Autodesk Inventor part; units mm, degrees
ref_plane "YZ Plane" through (0, 0, 0) normal (1, 0, 0) x (0, 1, 0)
ref_plane "XZ Plane" through (0, 0, 0) normal (0, 1, 0) x (-1, 0, 0)
ref_plane "XY Plane" through (0, 0, 0) normal (0, 0, 1) x (1, 0, 0)
sketch "Sketch1" plane through (0, 0, 0) normal (0, 0, 1) x (1, 0, 0)
  line L0 (0, 0) -> (22.5, 0)
  line L1 (22.5, 0) -> (22.5, 22.5)
  line L2 (22.5, 22.5) -> (0, 22.5)
  line L3 (0, 22.5) -> (0, 0)
  line L4 (0, 0) -> (20.5, 0)
  line L5 (20.5, 0) -> (20.5, 2)
  line L6 (20.5, 2) -> (0, 2)
  line L7 (0, 2) -> (0, 0)
  line L8 (22.5, 0) -> (20.5, 0)
  line L9 (20.5, 0) -> (20.5, 20.5)
  line L10 (20.5, 20.5) -> (22.5, 20.5)
  line L11 (22.5, 20.5) -> (22.5, 0)
  line L12 (22.5, 22.5) -> (2, 22.5)
  line L13 (2, 22.5) -> (2, 20.5)
  line L14 (2, 20.5) -> (22.5, 20.5)
  line L15 (22.5, 20.5) -> (22.5, 22.5)
  line L16 (0, 22.5) -> (2, 22.5)
  line L17 (2, 22.5) -> (2, 2)
  line L18 (2, 2) -> (0, 2)
  line L19 (0, 2) -> (0, 22.5)
  line L20 (2, 2) -> (20.5, 2)
  line L21 (20.5, 2) -> (20.5, 20.5)
  line L22 (20.5, 20.5) -> (2, 20.5)
  line L23 (2, 20.5) -> (2, 2)
  dimension "d0" = 22.5
  dimension "d1" = 22.5
  dimension "d2" = 20.5
  dimension "d3" = 2
  dimension "d4" = 2
  dimension "d5" = 20.5
  dimension "d6" = 20.5
  dimension "d7" = 2
  dimension "d8" = 2
  dimension "d9" = 20.5
  dimension "d10" = 18.5
  dimension "d11" = 18.5
extrude "Extrusion1" add sketch "Sketch1" along normal blind 69
sketch "Sketch2" plane through (0, 0, 0) normal (0, -1, 0) x (1, 0, 0)
  line L0 (0, 69) -> (22.5, 69)
  line L1 (22.5, 69) -> (20.5, 69)
  line L2 (20.5, 69) -> (20.5, 2)
  line L3 (20.5, 2) -> (22.5, 2)
  line L4 (22.5, 2) -> (22.5, 69)
  line L5 (20.5, 2) -> (2, 2)
  line L6 (2, 2) -> (2, 68)
  line L7 (2, 68) -> (20.5, 68)
  line L8 (20.5, 68) -> (20.5, 2)
  point P0 (0, 0)
  dimension "d14" = 2
  dimension "d15" = 67
  dimension "d16" = 18.5
  dimension "d17" = 66
extrude "Extrusion2" cut sketch "Sketch2" against normal blind 18.5 contours L2 L5 L6 L7
sketch "Sketch3" plane through (0, 0, 69) normal (0, 0, 1) x (1, 0, 0)
  line L0 (22.5, 22.5) -> (0, 22.5)
  line L1 (0, 0) -> (22.5, 0)
  line L2 (0, 22.5) -> (22.5, 22.5)
  line L3 (22.5, 22.5) -> (22.5, 0)
  line L4 (22.5, 0) -> (0, 0)
  line L5 (0, 0) -> (0, 22.5)
  dimension "d20" = 22.5
  dimension "d21" = 22.5
extrude "Extrusion3" add sketch "Sketch3" along normal blind 1
sketch "Sketch4" plane through (0, 18.5, 0) normal (0, -1, 0) x (1, 0, 0)
  point P0 (0, 0)
sketch "Sketch5" plane through (0, 18.5, 0) normal (0, -1, 0) x (1, 0, 0)
  line L0 (20.5, 2) -> (2, 2)
  line L1 (20.5, 68) -> (20.5, 2)
  line L2 (2, 2) -> (20.5, 2)
  line L3 (20.5, 2) -> (20.5, 68)
  line L4 (20.5, 68) -> (2, 68)
  line L5 (2, 68) -> (2, 2)
  point P0 (0, 0)
  dimension "d24" = 18.5
  dimension "d25" = 66
extrude "Extrusion4" cut sketch "Sketch5" against normal blind 2
properties part number "1-Battery-Case"
Can you work these out from the model? Positions are in its coordinate system, mm. A direction names the side the tool comes from. Coordinates: 2 decimals unless noted, no trailing zeros. Write each loop counter-clockwise with the first axis right and the second up, starting at its lowest first coordinate (ties: lowest second). Pieces come first, ordered by that corner, then holes. Notation, with made-up numbers: M 54.5,88.5 L 65.5,88.5 A19 cw 65.5,113.5 Z; hole C -26,72.5 d8. An arc over 180 degrees is marked long. Write item = value, one per line. Start each with the question number.
Q1. If we section it at A-A, the plane y = 3.25: Write out the boundary of the cut face in (x, z), then the cut area to 3 significant figures.
Q2. If we section it at C-C, the plane z = 30: Write out the boundary of the cut face in (x, y).
Q3. If we section it at B-B, the plane x = 2.75: Write out the boundary of the cut face in (y, z), then the cut area to 3 significant figures.
Q4. On a 3-axis mill with a long thin cutter (end or side, diameter ignored), from which of +Z, -Z, +X, -X, +Y, -Y can I reach the whole of each face in a straight line? I mean faces 1 (the face through (21, 0, 35)), 2 (the face through (2, 10, 35)). Say none if no direction works.
Q5. If I drill on L1, parallel to Z at x = 17.25, y = 15.5; L2, parallel to X at y = 17.5, z = 30.5; L3, parallel to Y at x = 2.25, z = 42.5, over which ranges is the centre line in solid material (lowest first)? Write a range as [from, to].
Q6. I'm going to push a flat-ended pin straight in: pin 1 (12 mm diameter, centred on x = 18.5, z = 34.5, fed in from -Y). Where does the tip first touch, or does it pass through?
Q7. Thinking about a two-plate mould opening in Z: for faces 3 (the face through (11, 10, 68)), 4 (the face through (11, 11, 0)), 5 (the face through (11, 11, 70)), 6 (the face through (22.5, 11, 35)), which applies, released by +Z, released by -Z, zero draft, split by the parting line, or undercut?
Check sheet entries:
q1.outline = M 0,0 L 22.5,0 L 22.5,70 L 0,70 Z; hole M 2,2 L 20.5,2 L 20.5,68 L 2,68 Z
q1.area = 354 mm²
q2.outline = M 0,0 L 2,0 L 2,20.5 L 20.5,20.5 L 20.5,0 L 22.5,0 L 22.5,22.5 L 0,22.5 Z
q3.outline = M 0,0 L 22.5,0 L 22.5,70 L 0,70 L 0,68 L 20.5,68 L 20.5,2 L 0,2 Z
q3.area = 222 mm²
q4.face_1 = +Z, -Z, +X, -X, -Y
q4.face_2 = -Y
q5.L1 = [0, 2], [68, 70]
q5.L2 = [0, 2], [20.5, 22.5]
q5.L3 = [20.5, 22.5]
q6.pin_1 = 0
q7.face_3 = undercut
q7.face_4 = released by -Z
q7.face_5 = released by +Z
q7.face_6 = zero draft
